Read the model definition and answer for the solid it produces. Units are mm, in the model's axes. Give positions to 0.01 mm unless a question says otherwise; leave off trailing zeros. Write each loop counter-clockwise with the first axis right and the second up, starting at its lowest first coordinate (ties: lowest second). Pieces come first, ordered by that corner, then holes. Notation, with made-up numbers: (29.5, 77.5) - (87.5, 77.5) arc R37 ccw to (87.5, 116.5) - close; hole circle Ø3 at (-7.75, -39.75). An arc over 180 degrees is marked (long way). Use CSV: the item, a comma, the result in double quotes. Start each with the question number.
from build123d import *

# Parameters (mm, degrees)
F1_DEPTH = 2.5
F2_COUNT = 4


with BuildPart() as f1:
    # F0 (on Front) → F1 (new body, symmetric)
    with BuildSketch(Plane.XZ):
        with BuildLine():
            ThreePointArc((18, 24), (17.0470416958, 29.7791322377), (14.2890700643, 34.946345358))
            ThreePointArc((14.2890700643, 34.946345358), (-4.1125794445, 31.1526624853), (-16.6488897576, 17.157889957))
            ThreePointArc((-16.6488897576, 17.157889957), (3.4871180339, 6.3410077349), (18, 24))
        make_face()
        with BuildLine():
            ThreePointArc((14.2890700643, 34.946345358), (7.967615209, 40.1405423664), (4.77e-08, 42))
            ThreePointArc((4.77e-08, 42), (-14.9525579748, 34.0210283908), (-16.6488897576, 17.157889957))
            ThreePointArc((-16.6488897576, 17.157889957), (-4.1125794445, 31.1526624853), (14.2890700643, 34.946345358))
        make_face()
        with BuildLine():
            ThreePointArc((40.8410037042, 5.1451568183), (40.1076678925, 11.7377562518), (37.9435125515, 18.0080497349))
            ThreePointArc((37.9435125515, 18.0080497349), (28.3069956895, 29.5365307848), (14.2890700643, 34.946345358))
            ThreePointArc((14.2890700643, 34.946345358), (17.0470416958, 29.7791322377), (18, 24))
            ThreePointArc((18, 24), (3.4871180339, 6.3410077349), (-16.6488897576, 17.157889957))
            Line((-16.6488897576, 17.157889957), (-10.2130597935, -16.2260015554))
            ThreePointArc((-10.2130597935, -16.2260015554), (10.3536707871, -24.8508846976), (31.1897226642, -16.8986549366))
            ThreePointArc((31.1897226642, -16.8986549366), (38.3224662635, -6.8868511438), (40.8410037042, 5.1451568183))
        make_face()
        with BuildLine():
            ThreePointArc((-5.3092368295, -41.6630772302), (4.7480675162, -41.730754305), (14.5331010068, -39.4054434707))
            Line((14.5331010068, -39.4054434707), (31.1897226642, -16.8986549366))
            ThreePointArc((31.1897226642, -16.8986549366), (10.3536707871, -24.8508846976), (-10.2130597935, -16.2260015554))
            Line((-10.2130597935, -16.2260015554), (-5.3092368295, -41.6630772302))
        make_face()
        with BuildLine():
            Line((9.3043480393, -46.4706479136), (14.5331010068, -39.4054434707))
            ThreePointArc((14.5331010068, -39.4054434707), (4.7480675162, -41.730754305), (-5.3092368295, -41.6630772302))
            Line((-5.3092368295, -41.6630772302), (-5.0224929571, -43.1504730102))
            ThreePointArc((-5.0224929571, -43.1504730102), (2.7091439762, -42.3586575491), (9.3043480393, -46.4706479136))
        make_face()
        with BuildLine():
            Line((2.6361842657, -55.4808154644), (9.3043480393, -46.4706479136))
            ThreePointArc((9.3043480393, -46.4706479136), (2.7091439762, -42.3586575491), (-5.0224929571, -43.1504730102))
            Line((-5.0224929571, -43.1504730102), (-2.982985598, -53.729791108))
            ThreePointArc((-2.982985598, -53.729791108), (0.1597548214, -51.0531040274), (3, -54.0488474071))
            ThreePointArc((3, -54.0488474071), (2.9076238406, -54.7875784822), (2.6361842657, -55.4808154644))
        make_face()
        with BuildLine():
            ThreePointArc((14.2890700643, 34.946345358), (28.3069956895, 29.5365307848), (37.9435125515, 18.0080497349))
            ThreePointArc((37.9435125515, 18.0080497349), (22.4461791063, 35.4988597497), (4.77e-08, 42))
            ThreePointArc((4.77e-08, 42), (7.967615209, 40.1405423664), (14.2890700643, 34.946345358))
        make_face()
    extrude(amount=F1_DEPTH, both=True)

    # F2: F1 ×4 about axis
    f2_axis = Axis((0, 0, -54.0488474071), (0, -1, 0))


with BuildPart() as f1_1:
    add(f1.part)
    for i in range(1, F2_COUNT):
        add(f1.part.rotate(f2_axis, i * 360 / F2_COUNT))


solid = f1_1.part
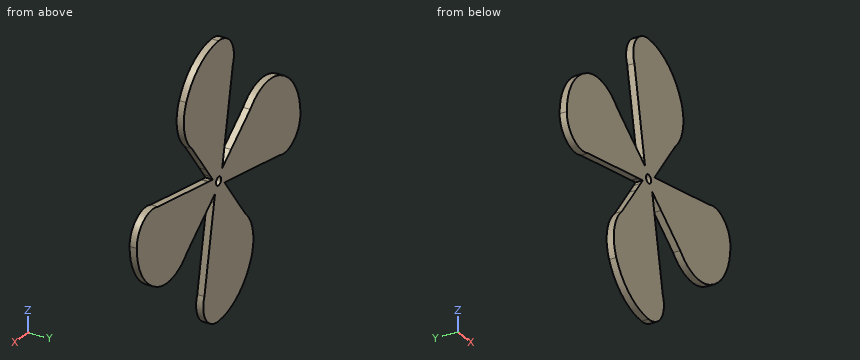
(1) Consider probe 1 along X at (y, z) = (1.1, -53.5); probe 2 along X at (y, z) = (-1.6, -52); probe 3 along Z at (x, y) = (32, 0.35). Determine where each line is inside the solid, lowest interval first.
(2) Given P1, Ø3, axis at y = 0.5, z = 20.5, coming from the +X side; P2, Ø3, axis at y = 2, z = -54.5, coming from the +X side; P3, Ø1.5, axis at x = -2, y = -0.5, coming from the -Z side, each flat-ended and moving along its own axis, determine where each tip first touches the part or whether it passes through.
(3) The part is cut by section A-A on x = 52. Write down the section's boundary in (y, z), plus the area to 3 significant figures.
(4) The part is cut by section B-B on z = -100. Write down the section's boundary in (x, y), plus the area to 3 significant figures.
Reported:
1,probe 1,"-96.05 to -2.95, 2.95 to 96.04"
1,probe 2,"-96 to -2.19, 2.19 to 95.93"
1,probe 3,"-81.43 to -44.96, -16.12 to 27.2"
2,P1,"x = 37.46"
2,P2,"x = 96.05"
2,P3,"z = -150.08"
3,outline,"(-2.5, -94.01) - (2.5, -94.01) - (2.5, -41.1) - (-2.5, -41.1) - close"
3,area,"265 mm²"
4,outline,"(-37.76, -2.5) - (11.78, -2.5) - (11.78, 2.5) - (-37.76, 2.5) - close"
4,area,"248 mm²"
